Answer from the drawing. Dimensions are ordinates in mm from the lowest x, y and z of the part. A direction names the side the tool comes from. Coordinates: 2 decimals unless noted, no trailing zeros. Write each loop counter-clockwise with the first axis right and the second up, starting at its lowest first coordinate (ties: lowest second). Pieces come first, ordered by that corner, then holes.
(1) Determine the mould class of the marked faces 1, 2 and 3 for opening direction Z: pulls with the +Z half, pulls with the -Z half, needs draft (parallel to the pull), parting line crosses it, or undercut.
(2) Given pin 1 (1.5 mm diameter, centred on x = 3, y = 0.5, fed in from +Z); pin 2 (0.5 mm diameter, centred on y = 3, z = 3.5, fed in from +X); pin 3 (0.7 mm diameter, centred on x = 5.5, y = 2.5, fed in from -Z), each flat-ended and moving along its own axis, determine where each tip first touches the part or whether it passes through.
(3) Which of the six approach directions +Z, -Z, +X, -X, +Y, -Y give full straight-line access (tool end or side, diameter ignored) to the marked faces 4 and 5?
(4) The part is cut by section D-D, the plane x = 6.75. Determine the outline of the cut face in (y, z).
(5) The part is cut by section A-A, the plane z = 4. Determine the outline of the cut face in (x, y).
(6) The part is cut by section C-C, the plane y = 2.6. Determine the outline of the cut face in (x, z).
(7) The part is cut by section B-B, the plane x = 4. Determine the outline of the cut face in (y, z).
(8) Straight lines are drawn through the part: line 1 along X through (y, z) = (3.35, 4); line 2 along Z through (x, y) = (4.75, 0.65); line 3 along X through (y, z) = (0.6, 5.75). For each, find the intervals that lie inside material, in ascending order.
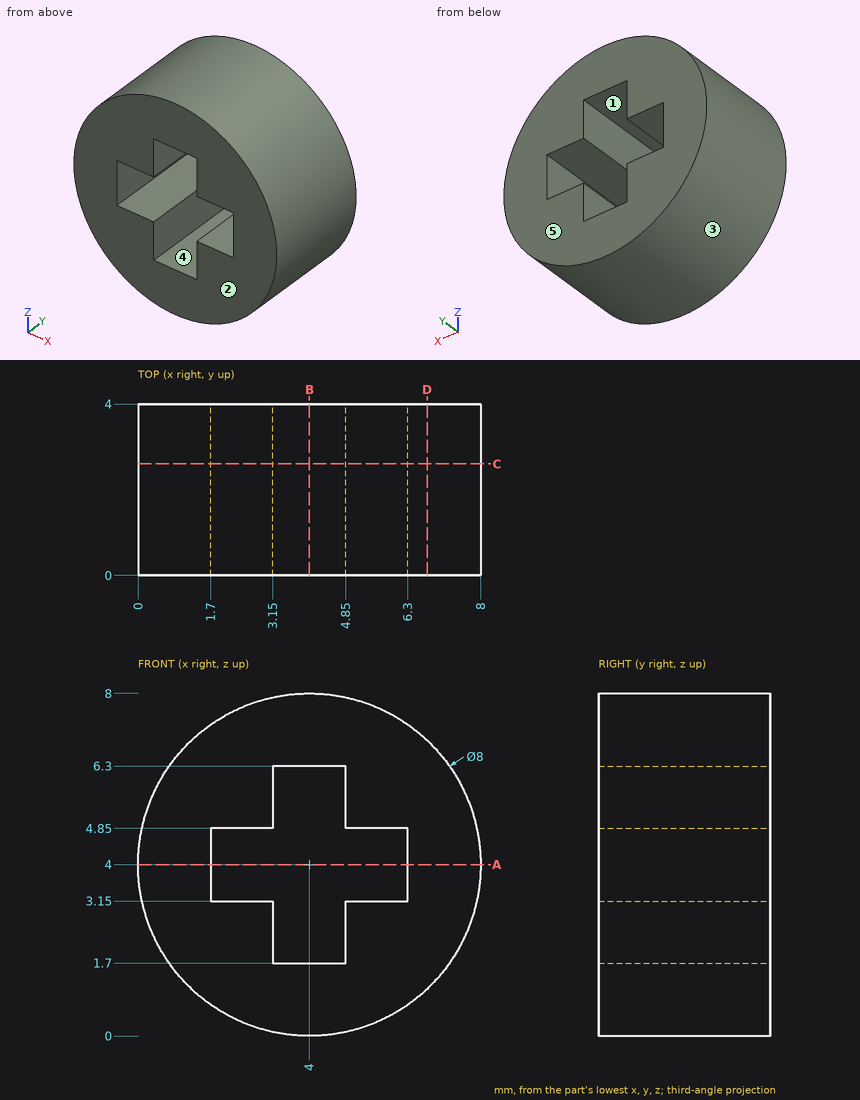
Computed:
1. face 1: undercut
1. face 2: needs draft
1. face 3: parting line crosses it
2. pin 1: stops at z = 7.99
2. pin 2: stops at x = 7.99
2. pin 3: stops at z = 0.17
3. face 4: +Y, -Y
3. face 5: +Z, -Z, +X, -X, +Y
4. outline: (0, 1.1) - (4, 1.1) - (4, 6.9) - (0, 6.9) - close
5. outline: (0, 0) - (1.7, 0) - (1.7, 4) - (0, 4) - close; (6.3, 0) - (8, 0) - (8, 4) - (6.3, 4) - close
6. outline: circle Ø8 at (4, 4); hole (1.7, 3.15) - (3.15, 3.15) - (3.15, 1.7) - (4.85, 1.7) - (4.85, 3.15) - (6.3, 3.15) - (6.3, 4.85) - (4.85, 4.85) - (4.85, 6.3) - (3.15, 6.3) - (3.15, 4.85) - (1.7, 4.85) - close
7. outline: (0, 0) - (4, 0) - (4, 1.7) - (0, 1.7) - close; (0, 6.3) - (4, 6.3) - (4, 8) - (0, 8) - close
8. line 1: x = 0 to 1.7, 6.3 to 8
8. line 2: z = 0.07 to 1.7, 6.3 to 7.93
8. line 3: x = 0.4 to 3.15, 4.85 to 7.6
